Part model, mm, in its own coordinate system. A direction names the side the tool comes from. Round coordinates to 2 decimals unless told otherwise and drop trailing zeros. Write each loop counter-clockwise with the first axis right and the second up, starting at its lowest first coordinate (ties: lowest second). Pieces come first, ordered by that corner, then holes. Notation, with made-up numbers: (-36.75, -39.5) -> (5.25, -39.5) arc R16 cw to (5.25, -32.5) -> close; hole circle Ø5 at (87, -36.5). An arc over 180 degrees is marked (long way). Use CSV: the item, a comma, the result in double quotes. Start each with the question number.
(1) Saw through at B-B (x = 36). Give the cut face in (y, z).
(2) Saw through at D-D (y = 35). Give the cut face in (x, z), plus the area to 3 significant figures.
(3) Saw through at A-A (y = 29). Give the cut face in (x, z).
(4) Probe line 1 (Y direction, x = 6, z = 7.5); line 2 (Y direction, x = 32.5, z = 9.5); line 3 (Y direction, x = 24, z = 1.3). List the from-to ranges inside material, lowest first. Write a range as [from, to].
(5) Saw through at C-C (z = 6.75). Count the separate pieces of the cut face and the enclosed holes in it, plus the area to 3 significant figures.
(6) Which spindle directions (+Z, -Z, +X, -X, +Y, -Y) get a long thin tool onto all of the face, cutting with end or side? Do faces 1 (the flat face through (90, 6, 4.5)), 2 (the flat face through (9, 14.75, 1)), 3 (the cylindrical face through (0.68, 0.64, 5.07)), 4 (the flat face through (98, 20, 2)). Say none if no direction does.
(7) Two-plate mould, pull along Y, no slides. Class faces 5 (the cylindrical face through (0.64, 39.32, 5.07)), 6 (the flat face through (65, 39, 10)), 7 (the cylindrical face through (8.1, 31.86, 5.58)): released by +Y, released by -Y, zero draft, split by the parting line, or undercut.
(8) Drop flat-ended pins along their axis: pin 1 (5.5 mm diameter, centred on x = 75.5, y = 33, fed in from +Z); pin 2 (3 mm diameter, centred on x = 73.5, y = 7, fed in from +Z); pin 3 (16 mm diameter, centred on x = 56, y = 20, fed in from +Z); pin 4 (3.5 mm diameter, centred on x = 90.125, y = 6, fed in from +Z). Give the stop position or say it passes through.
```python
from build123d import *

# Parameters (mm, degrees)
BODY_DEPTH          = 10
SKETCH10_W          = 75.5
SKETCH10_H          = 35.5
PCB_RECESS_DEPTH    = 7.75
SKETCH11_R          = 3
PCB_BOSS_DEPTH      = 6.75
FILLET2_R           = 2.25
SKETCH12_R          = 2
M3_INSERTS_DEPTH    = 5.5
FILLET3_R           = 2.25
SKETCH27_R          = 5
MAGNETS_DEPTH       = 1.75
SKETCH29_W          = 2
SKETCH29_H          = 7.75
SKETCH30_W          = 2.5
SKETCH30_H          = 20.5
HIROSE_MID_DEPTH    = 109.166538264
SKETCH31_R          = 2
CUT_EXTRUDE14_DEPTH = 5.5
SKETCH32_W          = 17.75
SKETCH32_H          = 6.5


with BuildPart() as part:
    # Sketch4 → body (new body)
    with BuildSketch(Plane.XY):
        Polygon((0, 40), (0, 25.25), (14.7, 25.25), (14.7, 14.75), (0, 14.75), (0, 0), (100, 0), (100, 40), align=None)
    extrude(amount=BODY_DEPTH)

    # Sketch10 → pcb-recess (cut)
    with BuildSketch(Plane.XY.offset(10)):
        with Locations((40, 20)):
            Rectangle(SKETCH10_W, SKETCH10_H)
    extrude(amount=-PCB_RECESS_DEPTH, mode=Mode.SUBTRACT)

    # Sketch11 → pcb-boss (add)
    with BuildSketch(Plane.XY.offset(2.25)):
        with Locations((6, 34)):
            Circle(SKETCH11_R)
        with BuildLine():
            ThreePointArc((6, 31), (3.878679656, 36.121320344), (9, 34))
            Line((9, 34), (9, 37.75))
            Line((9, 37.75), (2.25, 37.75))
            Line((2.25, 37.75), (2.25, 31))
            Line((2.25, 31), (6, 31))
        make_face()
        with BuildLine():
            Line((77.75, 37.75), (71, 37.75))
            Line((71, 37.75), (71, 34))
            ThreePointArc((71, 34), (74, 37), (77, 34))
            ThreePointArc((77, 34), (76.121320344, 31.878679656), (74, 31))
            Line((74, 31), (77.75, 31))
            Line((77.75, 31), (77.75, 37.75))
        make_face()
        with Locations((74, 34)):
            Circle(SKETCH11_R)
        with Locations((74, 6)):
            Circle(SKETCH11_R)
        with BuildLine():
            Line((77.75, 2.25), (77.75, 9))
            Line((77.75, 9), (74, 9))
            ThreePointArc((74, 9), (76.121320344, 8.121320344), (77, 6))
            ThreePointArc((77, 6), (74, 3), (71, 6))
            Line((71, 6), (71, 2.25))
            Line((71, 2.25), (77.75, 2.25))
        make_face()
        with Locations((6, 6)):
            Circle(SKETCH11_R)
        with BuildLine():
            Line((2.25, 2.25), (9, 2.25))
            Line((9, 2.25), (9, 6))
            ThreePointArc((9, 6), (3.878679656, 3.878679656), (6, 9))
            Line((6, 9), (2.25, 9))
            Line((2.25, 9), (2.25, 2.25))
        make_face()
    extrude(amount=PCB_BOSS_DEPTH)

    # Fillet2
    fillet2_edges = [part.edges().sort_by_distance(p)[0] for p in [
        (0, 14.75, 5),
        (0, 25.25, 5),
    ]]
    fillet(fillet2_edges, radius=FILLET2_R - 0.0001)  # a hair under: the kernel refuses the full size

    # Sketch12 → m3-inserts (cut)
    with BuildSketch(Plane.XY.offset(9)):
        with Locations((6, 34)):
            Circle(SKETCH12_R)
        with Locations((74, 34)):
            Circle(SKETCH12_R)
        with Locations((74, 6)):
            Circle(SKETCH12_R)
        with Locations((6, 6)):
            Circle(SKETCH12_R)
    extrude(amount=-M3_INSERTS_DEPTH, mode=Mode.SUBTRACT)

    # Fillet3
    fillet3_edges = [part.edges().sort_by_distance(p)[0] for p in [
        (0, 40, 5),
        (100, 40, 5),
        (100, 0, 5),
        (0, 0, 5),
    ]]
    fillet(fillet3_edges, radius=FILLET3_R)

    # Sketch27 → magnets (cut)
    with BuildSketch(Plane.XY.offset(2.25)):
        with Locations((24, 20)):
            Circle(SKETCH27_R)
        with Locations((56, 20)):
            Circle(SKETCH27_R)
    extrude(amount=-MAGNETS_DEPTH, mode=Mode.SUBTRACT)

    # Sketch29 → hirose-front (revolve, cut)
    with BuildSketch(Plane.XY.offset(10)):
        with Locations((99, 23.875)):
            Rectangle(SKETCH29_W, SKETCH29_H)
    revolve(axis=Axis((100, 20, 10), (-1, 0, 0)), mode=Mode.SUBTRACT)

    # Sketch30 → hirose-mid (cut, through all)
    with BuildSketch(Plane.XY.offset(10)):
        with Locations((96.75, 20)):
            Rectangle(SKETCH30_W, SKETCH30_H)
    extrude(amount=-HIROSE_MID_DEPTH, mode=Mode.SUBTRACT)

    # Sketch31 → Cut-Extrude14 (cut)
    with BuildSketch(Plane.XY.offset(10)):
        with Locations((90.125, 34)):
            Circle(SKETCH31_R)
        with Locations(Location((90.125, 6, 0), (0, 0, 180))):
            Circle(SKETCH31_R)
    extrude(amount=-CUT_EXTRUDE14_DEPTH, mode=Mode.SUBTRACT)

    # Sketch32 → hirose-back (revolve, cut)
    with BuildSketch(Plane.XY.offset(10)):
        with Locations((86.625, 23.25)):
            Rectangle(SKETCH32_W, SKETCH32_H)
    revolve(axis=Axis((77.75, 20, 10), (1, 0, 0)), mode=Mode.SUBTRACT)


solid = part.part
```
Answers:
1,outline,"(0, 0) -> (40, 0) -> (40, 10) -> (37.75, 10) -> (37.75, 2.25) -> (2.25, 2.25) -> (2.25, 10) -> (0, 10) -> close"
2,outline,"(0, 0) -> (100, 0) -> (100, 10) -> (91.86, 10) -> (91.86, 4.5) -> (88.39, 4.5) -> (88.39, 10) -> (77.75, 10) -> (77.75, 9) -> (75.73, 9) -> (75.73, 3.5) -> (72.27, 3.5) -> (72.27, 9) -> (71, 9) -> (71, 2.25) -> (9, 2.25) -> (9, 9) -> (7.73, 9) -> (7.73, 3.5) -> (4.27, 3.5) -> (4.27, 9) -> (2.25, 9) -> (2.25, 10) -> (0, 10) -> close"
2,area,"449 mm²"
3,outline,"(0, 0) -> (95.5, 0) -> (95.5, 10) -> (77.75, 10) -> (77.75, 2.25) -> (2.25, 2.25) -> (2.25, 10) -> (0, 10) -> close; (98, 0) -> (100, 0) -> (100, 10) -> (98, 10) -> close"
4,line 1,"y = [0, 4], [8, 9], [31, 32], [36, 40]"
4,line 2,"y = [0, 2.25], [37.75, 40]"
4,line 3,"y = [0, 15], [25, 40]"
5,separate pieces,"2"
5,enclosed holes,"6"
5,area,"1,110 mm²"
6,face 1,"+Z"
6,face 2,"+Z, -Z, -X"
6,face 3,"+Z, -Z, -X, -Y"
6,face 4,"+Z, -Z"
7,face 5,"released by +Y"
7,face 6,"zero draft"
7,face 7,"undercut"
8,pin 1,"stops at z = 10"
8,pin 2,"stops at z = 9"
8,pin 3,"stops at z = 2.25"
8,pin 4,"stops at z = 4.5"
